Build history of the part. All positions in model axes, mm. Round coordinates to 2 decimals unless told otherwise and drop trailing zeros. Loops run counter-clockwise (first coordinate to the right, second up) from the corner with the lowest first, then second, coordinate; pieces in that order, holes last. Notation, with made-up numbers: (-19, -39) -> (5, -39) arc R13 ccw to (5, -19) -> close; hole circle Ø1 at (45, 38.5). An arc over 180 degrees is marked (long way). Put each result on its own line as item: value. Start each with the question number.
Item 1: Cut at A-A, the plane x = -25.4. List the corners of the cut face in (y, z) (3 decimals).
Item 2: Drill centre lines: probe 1 along Z at (x, y) = (25, 0.15); probe 2 along Z at (x, y) = (26, 0.2). Where is each one in solid material? Low to high. Write a range as [from, to].
Item 3: Pull direction X, two halves, no side cores. Call faces 1 (the flat face through (31.75, 2, 1)), 2 (the flat face through (0, 2, 57.15)), 3 (the cylindrical face through (-26.051, 1.61, -52.405)), 4 (the cylindrical face through (24.749, 1.61, -52.405)): +X half, -X half, draft (parallel to the pull), parting line (faces both ways), or undercut.
```python
from build123d import *

# Parameters (mm, degrees)
SKETCH1_W           = 63.5
SKETCH1_H           = 114.3
BOSS_EXTRUDE1_DEPTH = 3.175
SKETCH2_R           = 1.7
CUT_EXTRUDE1_DEPTH  = 66.454301807


with BuildPart() as part:
    # Sketch1 → Boss-Extrude1 (new body)
    with BuildSketch(Plane(origin=(0, 0, 0), x_dir=(1, 0, 0), z_dir=(0, 1, 0))):
        Rectangle(SKETCH1_W, SKETCH1_H)
    extrude(amount=BOSS_EXTRUDE1_DEPTH)

    # Sketch2 → Cut-Extrude1 (cut, through all)
    with BuildSketch(Plane(origin=(0, 3.175, 0), x_dir=(1, 0, 0), z_dir=(0, 1, 0))):
        with Locations(Location((-25.4, 53.975, 0), (0, 0, 270))):
            Circle(SKETCH2_R)
        with Locations(Location((25.4, 53.975, 0), (0, 0, 270))):
            Circle(SKETCH2_R)
    cut_extrude1 = extrude(amount=-CUT_EXTRUDE1_DEPTH, mode=Mode.SUBTRACT)

    # Mirror1: Cut-Extrude1 across plane
    add(cut_extrude1.mirror(Plane.XY), mode=Mode.SUBTRACT)


solid = part.part
```
Reply:
1. outline: (0, -57.15) -> (3.175, -57.15) -> (3.175, -55.675) -> (0, -55.675) -> close; (0, -52.275) -> (3.175, -52.275) -> (3.175, 52.275) -> (0, 52.275) -> close; (0, 55.675) -> (3.175, 55.675) -> (3.175, 57.15) -> (0, 57.15) -> close
2. probe 1: z = [-57.15, -55.63], [-52.32, 52.32], [55.63, 57.15]
2. probe 2: z = [-57.15, -55.57], [-52.38, 52.38], [55.57, 57.15]
3. face 1: +X half
3. face 2: draft
3. face 3: undercut
3. face 4: undercut
